Model file for the job. Use its own axes, mm. A direction names the side the tool comes from. Give positions to 0.01 mm unless a question says otherwise; leave off trailing zeros. Write each loop counter-clockwise with the first axis right and the second up, starting at its lowest first coordinate (ties: lowest second). Pieces come first, ordered by that corner, then holes.
```python
from build123d import *


with BuildPart() as f1:
    # F0 (on Front) → F1 (revolve)
    with BuildSketch(Plane.XZ):
        with BuildLine():
            ThreePointArc((4.4, 3.3), (4.341421, 3.441421), (4.2, 3.5))
            Line((4.2, 3.5), (2.2, 3.5))
            Line((2.2, 3.5), (2.2, 0))
            Line((2.2, 0), (4.2, 0))
            ThreePointArc((4.2, 0), (4.341421, 0.058579), (4.4, 0.2))
            Line((4.4, 0.2), (4.4, 0.375))
            ThreePointArc((4.4, 0.375), (4.253553, 0.728553), (3.9, 0.875))
            Line((3.9, 0.875), (3.25, 0.875))
            Line((3.25, 0.875), (3.25, 2.625))
            Line((3.25, 2.625), (3.9, 2.625))
            ThreePointArc((3.9, 2.625), (4.253553, 2.771447), (4.4, 3.125))
            Line((4.4, 3.125), (4.4, 3.3))
        make_face()
    revolve(axis=Axis((0, 0, 1.683479), (0, 0, 1)))


solid = f1.part
```
1. Slice it at A-A, the plane y = 0. Write the cut outline in (x, z) (3 decimals), and give its area (3 significant figures).
Calculated:
outline: (-4.4, 0.2) arc R0.2 ccw to (-4.2, 0) - (-2.2, 0) - (-2.2, 3.5) - (-4.2, 3.5) arc R0.2 ccw to (-4.4, 3.3) - (-4.4, 3.125) arc R0.5 ccw to (-3.9, 2.625) - (-3.25, 2.625) - (-3.25, 0.875) - (-3.9, 0.875) arc R0.5 ccw to (-4.4, 0.375) - close; (2.2, 0) - (4.2, 0) arc R0.2 ccw to (4.4, 0.2) - (4.4, 0.375) arc R0.5 ccw to (3.9, 0.875) - (3.25, 0.875) - (3.25, 2.625) - (3.9, 2.625) arc R0.5 ccw to (4.4, 3.125) - (4.4, 3.3) arc R0.2 ccw to (4.2, 3.5) - (2.2, 3.5) - close
area: 11.1 mm2
2. Slice it at D-D, the plane z = 2.85. Write the cut outline in (x, y).
Calculated:
outline: circle Ø8.64 at (0, 0); hole circle Ø4.4 at (0, 0)
3. Probe probe 1 along Y at (x, z) = (0, 1.45); probe 2 along Z at (x, y) = (3.5, 0.25) (3 decimals); probe 3 along X at (y, z) = (0.25, 2.5). List the from-to ranges inside material, lowest first.
Calculated:
probe 1: y = -3.25 to -2.2, 2.2 to 3.25
probe 2: z = 0 to 0.875, 2.625 to 3.5
probe 3: x = -3.24 to -2.19, 2.19 to 3.24
4. Which spindle directions (+Z, -Z, +X, -X, +Y, -Y) get a long thin tool onto all of the face, cutting with end or side? Do faces 1 (the flat face through (-2, -2, 0)), 2 (the flat face through (2, 3, 2.625)). Say none if no direction does.
Calculated:
face 1: -Z, +X, -X, +Y, -Y
face 2: none
5. Pin check, flat tips, straight feed: P1, Ø1, axis at x = -1, z = 1, coming from the -Y side; P2, Ø1.5, axis at x = 2.5, z = 1, coming from the +Y side. Stop position of each tip, or through.
Calculated:
P1: stops at y = -4.3
P2: stops at y = 3.93
6. Slice it at C-C, the plane z = 2.25. Write the cut outline in (x, y).
Calculated:
outline: circle Ø6.5 at (0, 0); hole circle Ø4.4 at (0, 0)
7. Pull direction Z, two halves, no side cores. Call faces 3 (the flat face through (2, -2, 3.5)), 4 (the cylindrical face through (-2.579, -1.978, 1.762)), 5 (the cylindrical face through (2.1, 0.66, 1.73)), 6 (the flat face through (-2, 3, 0.875)): +Z half, -Z half, draft (parallel to the pull), parting line (faces both ways), or undercut.
Calculated:
face 3: +Z half
face 4: undercut
face 5: draft
face 6: undercut
